Input: part model. Units: mm. Frame: model coordinates. Round coordinates to 2 decimals unless told otherwise and drop trailing zeros. Loops run counter-clockwise (first coordinate to the right, second up) from the corner with the lowest first, then second, coordinate; pieces in that order, holes last.
(1) Cut plane C-C, the plane z = 3.3. Give the number of separate pieces and of enclosed holes in the cut face, and give its area (3 significant figures).
(2) Cut plane A-A, the plane x = 310. Output: boundary loops of the cut face in (y, z) (3 decimals), and give its area (3 significant figures).
(3) Cut plane B-B, the plane y = 165.1. Output: boundary loops of the cut face in (x, z), and give its area (3 significant figures).
(4) Cut plane D-D, the plane x = 124. Output: boundary loops of the cut face in (y, z) (3 decimals).
(5) Line query: line 1 (X direction, y = -89, z = 1.95); line 2 (X direction, y = -91.5, z = 1); line 3 (Y direction, x = 81, z = 3.85) (3 decimals). Output: solid intervals per line, ascending.
(6) First-contact query: pin 1 Ø1.3 at (y, z) = (-2, 2.5) entering from +X. Flat tip, straight axial feed; report the tip coordinate or a pass-through.
from build123d import *

# Parameters (mm, degrees)
PAD_DEPTH           = 4.318
POCKET_DEPTH        = 5.08
LINEARPATTERN_COUNT = 4
LINEARPATTERN_PITCH = 126.492


with BuildPart() as part:
    # Sketch → Pad (new body)
    with BuildSketch(Plane.XY):
        Polygon((0, 224.155), (566.42, 224.155), (566.42, 14.2875), (520.7, 14.2875), (520.7, -14.2875), (566.42, -14.2875), (566.42, -224.155), (0, -224.155), align=None)
    extrude(amount=PAD_DEPTH)

    # Sketch001 (on Face10 of Pad) → Pocket (cut)
    with BuildSketch(Plane.XY.offset(4.318)):
        with BuildLine():
            ThreePointArc((62.995513, 179.734615), (36.165385, 177.295513), (38.604487, 150.465385))
            Line((38.604487, 150.465385), (114.804487, 86.965385))
            ThreePointArc((114.804487, 86.965385), (141.634615, 89.404487), (139.195513, 116.234615))
            Line((62.995513, 179.734615), (139.195513, 116.234615))
        make_face()
        with BuildLine():
            ThreePointArc((139.195513, -116.234615), (141.634615, -89.404487), (114.804487, -86.965385))
            Line((114.804487, -86.965385), (38.604487, -150.465385))
            ThreePointArc((38.604487, -150.465385), (36.165385, -177.295513), (62.995513, -179.734615))
            Line((139.195513, -116.234615), (62.995513, -179.734615))
        make_face()
    pocket = extrude(amount=-POCKET_DEPTH, mode=Mode.SUBTRACT)

    # LinearPattern: Pocket ×4
    with Locations(*[(i * LINEARPATTERN_PITCH, 0, 0) for i in range(1, LINEARPATTERN_COUNT)]):
        add(pocket, mode=Mode.SUBTRACT)


solid = part.part
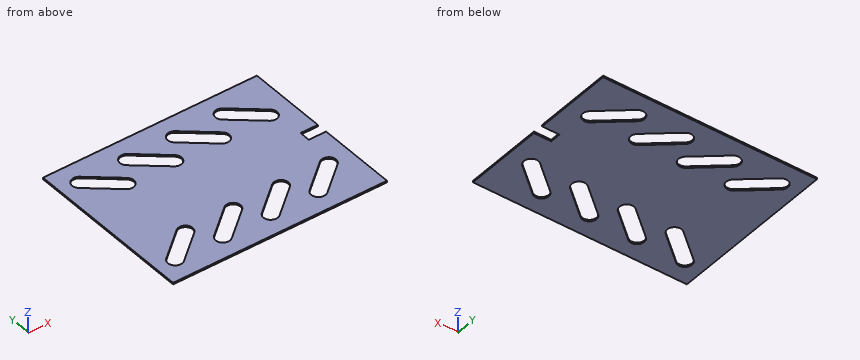
Reported:
1. separate pieces: 1
1. enclosed holes: 8
1. area: 213,000 mm2
2. outline: (-224.155, 0) - (-183.107, 0) - (-183.107, 4.318) - (-224.155, 4.318) - close; (-135.122, 0) - (135.122, 0) - (135.122, 4.318) - (-135.122, 4.318) - close; (183.107, 0) - (224.155, 0) - (224.155, 4.318) - (183.107, 4.318) - close
2. area: 1,520 mm2
3. outline: (0, 0) - (31.75, 0) - (31.75, 4.32) - (0, 4.32) - close; (80.56, 0) - (158.24, 0) - (158.24, 4.32) - (80.56, 4.32) - close; (207.05, 0) - (284.73, 0) - (284.73, 4.32) - (207.05, 4.32) - close; (333.54, 0) - (411.23, 0) - (411.23, 4.32) - (333.54, 4.32) - close; (460.03, 0) - (566.42, 0) - (566.42, 4.32) - (460.03, 4.32) - close
3. area: 1,600 mm2
4. outline: (-224.155, 0) - (-128.898, 0) - (-128.898, 4.318) - (-224.155, 4.318) - close; (-82.788, 0) - (82.788, 0) - (82.788, 4.318) - (-82.788, 4.318) - close; (128.898, 0) - (224.155, 0) - (224.155, 4.318) - (128.898, 4.318) - close
5. line 1: x = 0 to 112.36, 141.29 to 238.85, 267.78 to 365.35, 394.27 to 491.84, 520.76 to 566.42
5. line 2: x = 0 to 109.36, 143.15 to 235.85, 269.64 to 362.35, 396.14 to 488.84, 522.63 to 566.42
5. line 3: y = -224.155 to -164.731, -115.136 to 115.136, 164.731 to 224.155
6. pin 1: stops at x = 520.7
